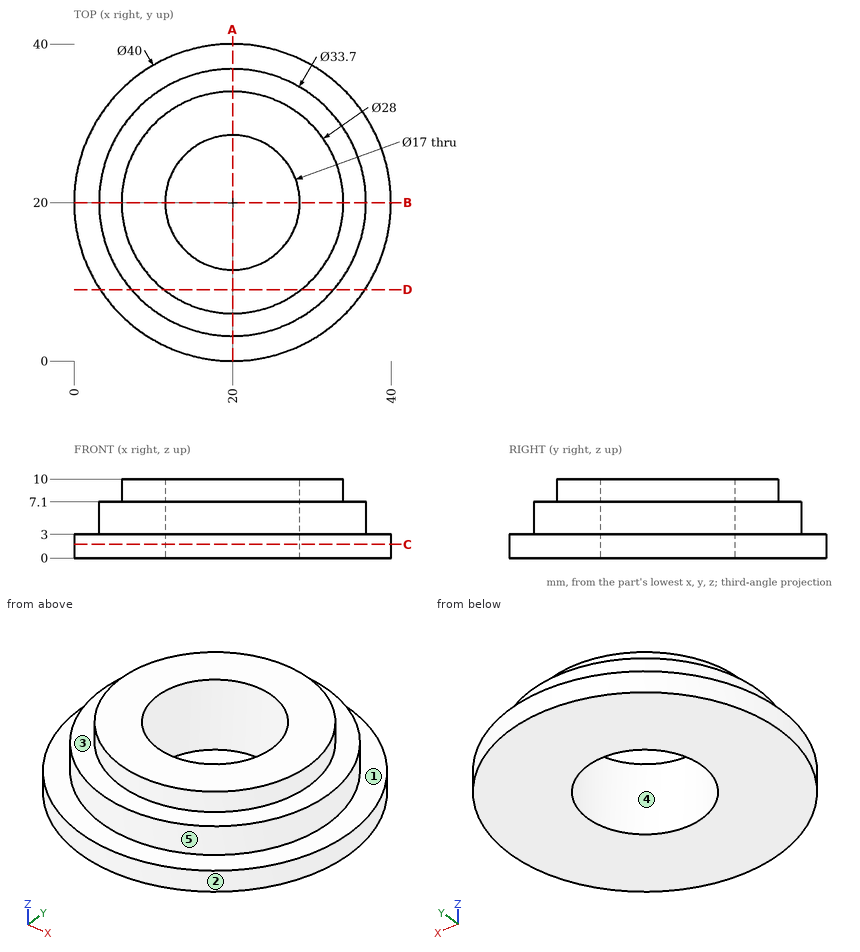
For this review, use the dimensioned drawing (mm, ordinates from the lowest corner) and the shaded views. A direction names the side the tool comes from. Give positions to 0.01 mm unless a question says otherwise; leave off trailing zeros. Order: outer loops, then holes, each group sorted by start corner. A loop starts at its lowest first (then second) coordinate and runs counter-clockwise, first axis right, second up. Notation, with made-up numbers: M -7.5,-9 L 23.5,-9 A24 ccw 23.5,11 Z; hole C 84.25,1.25 d10. An arc over 180 degrees is marked long. Use one line per item in the form item = value. Start each with the question number.
Item 1: To check wall thickness, follow line 1 along Y through (x, z) = (20, 7); line 2 along Y through (x, z) = (20, 7.25); line 3 along Z through (x, y) = (34, 14). State the ranges of each line that lie inside material, in increasing order. Write a range as from..to.
Item 2: For the marked faces 1 and 2, list the 3-axis set-ups (+Z, -Z, +X, -X, +Y, -Y) from which the entire face can be reached by the end or side of a thin tool; tool diameter is ignored.
Item 3: Insertion check: pin 1 Ø5 at (x, z) = (17, 1.5) entering from -Y; pin 2 Ø6 at (y, z) = (12, 4) entering from -X; pin 3 Ø3 at (x, y) = (35, 29) entering from +Z. Each pin has a flat end and moves straight along its axis. Give the tip position at first contact, or say it passes through.
Item 4: We need section A-A on x = 20. Give the boundary of the cut face in (y, z).
Item 5: We need section C-C on z = 1.75. Give the boundary of the cut face in (x, y).
Item 6: We need section D-D on y = 9. Give the boundary of the cut face in (x, z).
Item 7: The part is to be moulded in two halves that separate along Y. For the marked faces 3, 4 and 5, say which applies: pulls with the +Y half, pulls with the -Y half, needs draft (parallel to the pull), parting line crosses it, or undercut.
Completed:
q1.line_1 = 3.15..11.5, 28.5..36.85
q1.line_2 = 6..11.5, 28.5..34
q1.line_3 = 0..7.1
q2.face_1 = +Z
q2.face_2 = +Z, -Z
q3.pin_1 = 0.01
q3.pin_2 = 0.68
q3.pin_3 = 7.1
q4.outline = M 0,0 L 11.5,0 L 11.5,10 L 6,10 L 6,7.1 L 3.15,7.1 L 3.15,3 L 0,3 Z; M 28.5,0 L 40,0 L 40,3 L 36.85,3 L 36.85,7.1 L 34,7.1 L 34,10 L 28.5,10 Z
q5.outline = C 20,20 d40; hole C 20,20 d17
q6.outline = M 3.3,0 L 36.7,0 L 36.7,3 L 32.76,3 L 32.76,7.1 L 28.66,7.1 L 28.66,10 L 11.34,10 L 11.34,7.1 L 7.24,7.1 L 7.24,3 L 3.3,3 Z
q7.face_3 = needs draft
q7.face_4 = undercut
q7.face_5 = parting line crosses it
